```python
from build123d import *

# Parameters (mm, degrees)
SKETCH1_W            = 36
SKETCH1_H            = 110
BOSS_EXTRUDE1_DEPTH  = 1
M3_CLEARANCE_HOLE1_D = 3.4
M4_CLEARANCE_HOLE1_D = 4.5
M3_CLEARANCE_HOLE2_D = 3.4


with BuildPart() as part:
    # Sketch1 → Boss-Extrude1 (new body)
    with BuildSketch(Plane(origin=(0, 0, 0), x_dir=(0, 0, -1), z_dir=(1, 0, 0))):
        with Locations((0, -55)):
            Rectangle(SKETCH1_W, SKETCH1_H)
    extrude(amount=BOSS_EXTRUDE1_DEPTH)

    # M3 Clearance Hole1 (through all)
    with Locations(Plane.ZY):
        with Locations((-10, -10), (10, -10)):
            Hole(M3_CLEARANCE_HOLE1_D / 2)

    # M4 Clearance Hole1 (through all)
    with Locations(Plane.ZY):
        with Locations((-13, -19), (13, -19)):
            Hole(M4_CLEARANCE_HOLE1_D / 2)

    # M3 Clearance Hole2 (through all)
    with Locations(Plane(origin=(1, 0, 0), x_dir=(0, 0, -1), z_dir=(1, 0, 0))):
        with Locations((6, -104), (-6, -104), (6, -94), (-6, -94), (6, -84), (-6, -84), (6, -74), (-6, -74), (6, -64), (-6, -64), (6, -54), (-6, -54), (6, -44), (-6, -44), (6, -34), (-6, -34)):
            Hole(M3_CLEARANCE_HOLE2_D / 2)


solid = part.part
```
The listing builds one solid part. Answer for the finished solid, in the listing's coordinates (mm). Give positions to 0.01 mm unless a question says otherwise; leave off trailing zeros. Order: outer loops, then holes, each group sorted by start corner. A loop starts at its lowest first (then second) coordinate and runs counter-clockwise, first axis right, second up. Notation, with made-up numbers: (-6.75, 62) - (39.25, 62) arc R24 ccw to (39.25, 75) - close; hole circle Ø11 at (-23, 34). An arc over 180 degrees is marked (long way). Use one line per item in the form item = value. Start each with the question number.
(1) A cutting plane is placed at D-D, the plane y = -19. Write down the section's boundary in (x, z).
(2) Flat-ended cylindrical pins translate along their axes: pin 1 Ø10 at (y, z) = (-48, 14) entering from -X; pin 2 Ø3 at (y, z) = (-84, 6) entering from +X. Find the tip coordinate at first contact, or state that the pin passes through.
(3) A cutting plane is placed at B-B, the plane y = -104. Write down the section's boundary in (x, z).
(4) Consider line 1 (Z direction, x = 0.65, y = -84); line 2 (Y direction, x = 0.6, z = -13); line 3 (Z direction, x = 0.3, y = -93). Determine where each line is inside the solid, lowest interval first. Write a range as from..to.
(5) The mould has two halves that part along Z. Classify faces 1 (the cylindrical face through (0.49, -105.66, 5.63)), 2 (the flat face through (0, -54, 0)): released by +Z, released by -Z, zero draft, split by the parting line, or undercut.
(6) A cutting plane is placed at A-A, the plane x = 0.6. State how many separate pieces and enclosed holes the cut face has, then the cut area to 3 significant figures.
Ans:
q1.outline = (0, -18) - (1, -18) - (1, -15.25) - (0, -15.25) - close; (0, -10.75) - (1, -10.75) - (1, 10.75) - (0, 10.75) - close; (0, 15.25) - (1, 15.25) - (1, 18) - (0, 18) - close
q2.pin_1 = 0
q2.pin_2 = through
q3.outline = (0, -18) - (1, -18) - (1, -7.7) - (0, -7.7) - close; (0, -4.3) - (1, -4.3) - (1, 4.3) - (0, 4.3) - close; (0, 7.7) - (1, 7.7) - (1, 18) - (0, 18) - close
q4.line_1 = -18..-7.7, -4.3..4.3, 7.7..18
q4.line_2 = -110..-21.25, -16.75..0
q4.line_3 = -18..-7.37, -4.63..4.63, 7.37..18
q5.face_1 = undercut
q5.face_2 = zero draft
q6.separate_pieces = 1
q6.enclosed_holes = 20
q6.area = 3,760 mm^2
